For this review, take the finished solid that the model builds, in its own axes (mm). A direction names the side the tool comes from. Give positions to 0.01 mm unless a question says otherwise; leave off trailing zeros. Write each loop counter-clockwise with the first axis right and the second up, starting at its lowest first coordinate (ties: lowest second). Pieces come first, ordered by that corner, then holes.
1) Wall thickness on line 1 along Z through (x, y) = (11.75, -1); line 2 along Z through (x, y) = (11.5, -13); line 3 along X through (y, z) = (4, 7.25): over which ranges is each line inside the solid? List them lowest first.
2) Draft analysis for pull direction Z (two halves, no side actions). For faces 1 (the face through (11.2, -0.4, 6.3)), 2 (the face through (0, 0, 0)), 3 (the face through (6, 0, -10)), state which applies: pulls with the +Z half, pulls with the -Z half, needs draft (parallel to the pull), parting line crosses it, or undercut.
3) We need section B-B on z = 7.75. Give the boundary of the cut face in (x, y), and give its area (3 significant figures).
4) We need section A-A on y = -8.5. Give the boundary of the cut face in (x, z).
5) Machinability: for faces 4 (the face through (11.2, -0.4, -7.7)), 5 (the face through (6, 30, 0)), which of the approach directions +Z, -Z, +X, -X, +Y, -Y give a long, thin tool a straight path to every point of the face, cutting with its end or side? Answer none if there is none.
from build123d import *

# Parameters (mm, degrees)
F0_W     = 60
F0_H     = 20
F1_DEPTH = 12
F3_DEPTH = 60.001


with BuildPart() as f1:
    # F0 (on Right) → F1 (new body)
    with BuildSketch(Plane.YZ):
        Rectangle(F0_W, F0_H)
    extrude(amount=F1_DEPTH)

    # F2 (on face) → F3 (cut, through all)
    with BuildSketch(Plane.XZ.offset(30)):
        Polygon((12, 8.5), (10.5, 7), (12, 5.5), align=None)
        Polygon((12, -8.5), (12, -5.5), (10.5, -7), align=None)
    extrude(amount=-F3_DEPTH, mode=Mode.SUBTRACT)


solid = f1.part
Results list:
1. line 1: z = -10 to -8.25, -5.75 to 5.75, 8.25 to 10
1. line 2: z = -10 to -8, -6 to 6, 8 to 10
1. line 3: x = 0 to 10.75
2. face 1: undercut
2. face 2: needs draft
2. face 3: pulls with the -Z half
3. outline: (0, -30) - (11.25, -30) - (11.25, 30) - (0, 30) - close
3. area: 675 mm2
4. outline: (0, -10) - (12, -10) - (12, -8.5) - (10.5, -7) - (12, -5.5) - (12, 5.5) - (10.5, 7) - (12, 8.5) - (12, 10) - (0, 10) - close
5. face 4: +X, +Y, -Y
5. face 5: +Z, -Z, +X, -X, +Y
